```python
from build123d import *

# Parameters (mm, degrees)
ESBO_O1_R                = 25
ESBO_O1_R_2              = 22
RESSALTO_EXTRUS_O1_DEPTH = 240
ESBO_O2_R                = 2.5
CORTE_EXTRUS_O1_DEPTH    = 243.590189414


with BuildPart() as part:
    # Esboço1 → Ressalto-extrusão1 (new body)
    with BuildSketch(Plane(origin=(0, 0, 0), x_dir=(1, 0, 0), z_dir=(0, 1, 0))):
        with Locations(Location((0, 0, 0), (0, 0, 270))):
            Circle(ESBO_O1_R)
        with Locations(Location((0, 0, 0), (0, 0, 270))):
            Circle(ESBO_O1_R_2, mode=Mode.SUBTRACT)
    extrude(amount=RESSALTO_EXTRUS_O1_DEPTH)

    # Esboço2 → Corte-extrusão1 (cut, symmetric)
    with BuildSketch(Plane.XY):
        with Locations((0, 15)):
            Circle(ESBO_O2_R)
    corte_extrus_o1 = extrude(amount=CORTE_EXTRUS_O1_DEPTH, both=True, mode=Mode.SUBTRACT)

    # Espelhar1: Corte-extrusão1 across plane
    add(corte_extrus_o1.mirror(Plane(origin=(0, 120, 0), x_dir=(0, 0, 1), z_dir=(0, -1, 0))), mode=Mode.SUBTRACT)


solid = part.part
```
The model under review builds one solid part; all positions refer to its coordinate system, in mm. Round coordinates to 2 decimals unless told otherwise and drop trailing zeros. Write each loop counter-clockwise with the first axis right and the second up, starting at its lowest first coordinate (ties: lowest second). Pieces come first, ordered by that corner, then holes. Notation, with made-up numbers: (78, -19.75) - (130, -19.75) arc R20 ccw to (130, -4.75) - close; hole circle Ø2 at (62.25, 74.5). An arc over 180 degrees is marked (long way). Answer as CSV lines item,"result". Start each with the question number.
(1) We need section B-B on x = 0. State the section outline as (y, z) points, plus the area to 3 significant figures.
(2) To check wall thickness, follow line 1 (Y direction, x = 0, z = 23.15); line 2 (X direction, y = 177.5, z = 0); line 3 (Z direction, x = -0.5, y = 154) (3 decimals). State the ranges of each line that lie inside material, in increasing order.
(3) We need section C-C on x = 19.5. State the section outline as (y, z) points.
(4) For pin 1 Ø5 at (x, y) = (10, 82.5) entering from +Z; pin 2 Ø1.5 at (y, z) = (198, -6) entering from -X; pin 3 Ø10 at (x, y) = (-6, 148.5) entering from +Z; pin 4 Ø3 at (x, y) = (0, 15) entering from -Z, all flat-tipped, find the tip position at first contact; note any pin that passes through.
(5) We need section A-A on z = 0. State the section outline as (x, y) points.
(6) We need section D-D on y = 23.5. State the section outline as (x, z) points.
(7) Draft analysis for pull direction X (two halves, no side actions). For faces 1 (the cylindrical face through (-0.33, 222.52, 23.45)), 2 (the cylindrical face through (7.509, 118.32, 23.846)), 3 (the flat face through (-22.1, 240, 1.7)), 4 (the cylindrical face through (-0.33, 222.52, -23.41)), state which applies: pulls with the +X half, pulls with the -X half, needs draft (parallel to the pull), parting line crosses it, or undercut.
Worked answers:
1,outline,"(0, -25) - (12.5, -25) - (12.5, -22) - (0, -22) - close; (0, 22) - (12.5, 22) - (12.5, 25) - (0, 25) - close; (17.5, -25) - (222.5, -25) - (222.5, -22) - (17.5, -22) - close; (17.5, 22) - (222.5, 22) - (222.5, 25) - (17.5, 25) - close; (227.5, -25) - (240, -25) - (240, -22) - (227.5, -22) - close; (227.5, 22) - (240, 22) - (240, 25) - (227.5, 25) - close"
1,area,"1,380 mm²"
2,line 1,"0 to 12.5, 17.5 to 222.5, 227.5 to 240"
2,line 2,"-25 to -22, 22 to 25"
2,line 3,"-24.995 to -21.994, 21.994 to 24.995"
3,outline,"(0, -15.64) - (240, -15.64) - (240, -10.19) - (0, -10.19) - close; (0, 10.19) - (240, 10.19) - (240, 15.64) - (0, 15.64) - close"
4,pin 1,"z = 23.85"
4,pin 2,"x = -24.44"
4,pin 3,"z = 24.98"
4,pin 4,"through"
5,outline,"(-25, 0) - (-22, 0) - (-22, 240) - (-25, 240) - close; (22, 0) - (25, 0) - (25, 240) - (22, 240) - close"
6,outline,"circle Ø50 at (0, 0); hole circle Ø44 at (0, 0)"
7,face 1,"undercut"
7,face 2,"parting line crosses it"
7,face 3,"needs draft"
7,face 4,"undercut"
